```python
from build123d import *

# Parameters (mm, degrees)
F0_W     = 68.58
F0_H     = 4.990084
F2_DEPTH = 10.414


with BuildPart() as f1:
    # F0 (on Top) → F1 (revolve)
    with BuildSketch(Plane.XY):
        Polygon((-3.261477, 16.393739), (0, 16.393739), (0, 19.904292), (-10.727971, 19.904292), align=None)
        with BuildLine():
            ThreePointArc((-3.261477, -35.100376), (-1.675796, -34.524032), (0, -34.328411))
            Line((0, -34.328411), (0, 16.393739))
            Line((0, 16.393739), (-3.261477, 16.393739))
            Line((-3.261477, 16.393739), (-3.261477, -35.100376))
        make_face()
        with BuildLine():
            Line((0, -48.879802), (0, -34.328411))
            ThreePointArc((0, -34.328411), (-1.675796, -34.524032), (-3.261477, -35.100376))
            ThreePointArc((-3.261477, -35.100376), (-7.080074, -43.279902), (0, -48.879802))
        make_face()
    revolve(axis=Axis((0, -8.967336, 0), (0, -1, 0)))

    # F0 (on Top) → F2 (join, symmetric)
    with BuildSketch(Plane.XY):
        Polygon((-10.727971, 19.904292), (0, 19.904292), (0, 24.894376), (-68.58, 24.894376), (-68.58, 19.904292), align=None)
        with Locations((34.29, 22.399334)):
            Rectangle(F0_W, F0_H)
    extrude(amount=F2_DEPTH, both=True)


solid = f1.part
```
Part model, mm, in its own coordinate system. A direction names the side the tool comes from. Round coordinates to 2 decimals unless told otherwise and drop trailing zeros. Write each loop counter-clockwise with the first axis right and the second up, starting at its lowest first coordinate (ties: lowest second). Pieces come first, ordered by that corner, then holes.
Item 1: Probe L1, parallel to Y at x = -19, z = 5.5; L2, parallel to Z at x = -13, y = 21; L3, parallel to X at y = -18, z = -1. List the from-to ranges inside material, lowest first.
Results:
L1: y = 19.9 to 24.89
L2: z = -10.41 to 10.41
L3: x = -3.1 to 3.1
Item 2: Which spindle directions (+Z, -Z, +X, -X, +Y, -Y) get a long thin tool onto all of the face, cutting with end or side? Do faces 1 (the flat face through (68.58, 22, 0)), 2 (the conical face through (0.786, 16.564, 3.538)). Say none if no direction does.
Results:
face 1: +Z, -Z, +X, +Y, -Y
face 2: none
Item 3: Cut at B-B, the plane y = -23. Give the cut face in (x, z), plus the area to 3 significant figures.
Results:
outline: circle Ø6.52 at (0, 0)
area: 33.4 mm2
Item 4: Drop flat-ended pins along their axis: pin 1 Ø1.5 at (y, z) = (-8, -1) entering from +X; pin 2 Ø12 at (y, z) = (-12.5, -1) entering from -X; pin 3 Ø3 at (y, z) = (-38.5, -7.5) entering from -X. Give the stop position or say it passes through.
Results:
pin 1: stops at x = 3.25
pin 2: stops at x = -3.26
pin 3: stops at x = -3.03
Item 5: Two-plate mould, pull along Y, no slides. Class faces 3 (the cylindrical face through (-3.11, -9.71, -0.98)), 4 (the flat face through (-36, 19.904, 0)), 5 (the flat face through (-1, 22, 10.414)): +Y half, -Y half, draft (parallel to the pull), parting line (faces both ways), or undercut.
Results:
face 3: undercut
face 4: -Y half
face 5: draft
Item 6: Cut at A-A, the plane x = -14.5. Give the cut face in (y, z), plus the area to 3 significant figures.
Results:
outline: (19.9, -10.41) - (24.89, -10.41) - (24.89, 10.41) - (19.9, 10.41) - close
area: 104 mm2
